Input: dimensioned drawing with shaded views. Units: mm. Origin: part minimum x, y, z. A direction names the side the tool comes from. Round coordinates to 2 decimals unless told otherwise and drop trailing zeros. Loops run counter-clockwise (first coordinate to the right, second up) from the corner with the lowest first, then second, coordinate; pieces in that order, holes last. Notation, with made-up numbers: (22.5, 20.5) - (71.5, 20.5) arc R7 ccw to (71.5, 24.5) - close; hole circle Ø6 at (-0.75, 29). An arc over 180 degrees is marked (long way). Write each question's results on one line, items separated by ' | '.
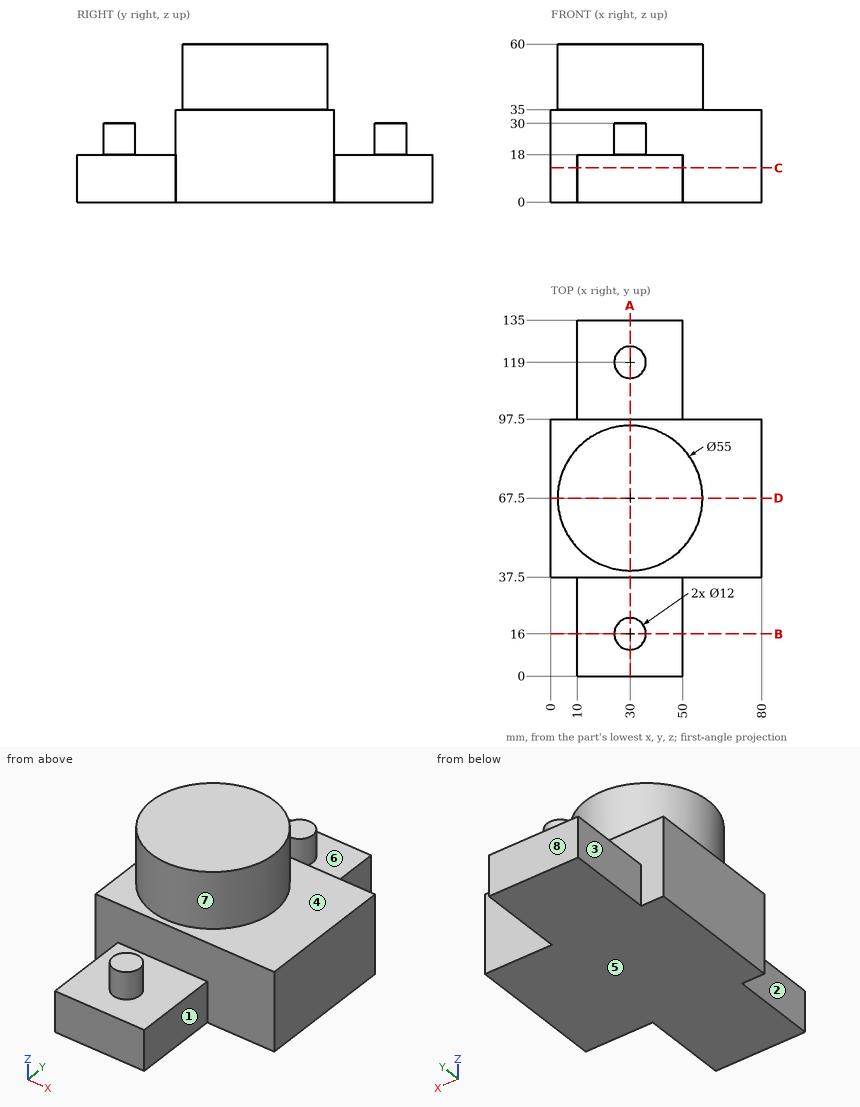
1. Contact query for flat-ended pins moving along their axis: pin 1 (1 mm diameter, centred on x = 57, z = 27.5, fed in from -Y); pin 2 (6 mm diameter, centred on x = 34.5, z = 41.5, fed in from +Y); pin 3 (13 mm diameter, centred on x = 32.5, y = 15, fed in from +Z); pin 4 (10.5 mm diameter, centred on x = 35, z = 18.5, fed in from -Y). Output: stop coordinate, or through.
Answer:
pin 1: y = 37.5 | pin 2: y = 94.96 | pin 3: z = 30 | pin 4: y = 0
2. Section query A-A, the plane x = 30. Output: boundary loops of the cut face in (y, z), plus the area to 3 significant figures.
Answer:
outline: (0, 0) - (135, 0) - (135, 18) - (125, 18) - (125, 30) - (113, 30) - (113, 18) - (97.5, 18) - (97.5, 35) - (95, 35) - (95, 60) - (40, 60) - (40, 35) - (37.5, 35) - (37.5, 18) - (22, 18) - (22, 30) - (10, 30) - (10, 18) - (0, 18) - close | area: 5,110 mm^2
3. Section query C-C, the plane z = 13. Output: boundary loops of the cut face in (x, y), plus the area to 3 significant figures.
Answer:
outline: (0, 37.5) - (10, 37.5) - (10, 0) - (50, 0) - (50, 37.5) - (80, 37.5) - (80, 97.5) - (50, 97.5) - (50, 135) - (10, 135) - (10, 97.5) - (0, 97.5) - close | area: 7,800 mm^2
4. Section query D-D, the plane y = 67.5. Output: boundary loops of the cut face in (x, z), plus the area to 4 significant figures.
Answer:
outline: (0, 0) - (80, 0) - (80, 35) - (57.5, 35) - (57.5, 60) - (2.5, 60) - (2.5, 35) - (0, 35) - close | area: 4,175 mm^2
5. Mould query, pull axis Y, two halves, no side actions, for the marked faces 5, 6, 7 and 8. Classes: pulls with the +Y half, pulls with the -Y half, needs draft (parallel to the pull), parting line crosses it, or undercut.
Answer:
face 5: needs draft | face 6: undercut | face 7: parting line crosses it | face 8: pulls with the +Y half
6. Section query B-B, the plane y = 16. Output: boundary loops of the cut face in (x, z).
Answer:
outline: (10, 0) - (50, 0) - (50, 18) - (36, 18) - (36, 30) - (24, 30) - (24, 18) - (10, 18) - close
7. Line query: line 1 (X direction, y = 29, z = 7.5); line 2 (X direction, y = 119.5, z = 24.5); line 3 (Y direction, x = 42, z = 21). Output: solid intervals per line, ascending. Write a range as [from, to].
Answer:
line 1: [10, 50] | line 2: [24.02, 35.98] | line 3: [37.5, 97.5]
8. Set-up query: the marked faces 1, 2, 3 and 4. Return all of +Z, -Z, +X, -X, +Y, -Y with unobstructed straight access to the full face (end or side cutting, diameter ignored); none if empty.
Answer:
face 1: +Z, -Z, +X, -Y | face 2: +Z, -Z, -X, -Y | face 3: +Z, -Z, -X, +Y | face 4: +Z
